For this review, take the finished solid that the model builds, in its own axes (mm). Face numbers are marked on the shaded views. A direction names the side the tool comes from. Give positions to 0.01 mm unless a question says otherwise; leave off trailing zeros. Loops run counter-clockwise (first coordinate to the right, second up) from the corner with the lowest first, then second, coordinate; pieces in that order, holes last. Notation, with made-up numbers: (22.25, -18) -> (77.25, -18) arc R35 ccw to (77.25, 14) -> close; hole circle Ø4 at (-34, 48.25). An arc over 180 degrees is marked (long way). One line per question, with ' | ' between items. Start each with the question number.
(1) Consider section A-A (y = 11.5). Write out the cut boundary in (x, z), and give its area (3 significant figures).
(2) Wall thickness on probe 1 along Z at (x, y) = (53.5, -22); probe 2 along Z at (x, y) = (6, -6.5): over which ranges is each line inside the solid? List them lowest first.
(3) Tool access review of the marked faces 1 and 2: name each direction out of +Z, -Z, +X, -X, +Y, -Y from which nothing blocks a thin tool from reaching the whole face with its end or side.
(4) Consider section B-B (z = 31.5). Write out the cut boundary in (x, y).
(5) Consider section C-C (x = 35.5). Write out the cut boundary in (y, z), and give its area (3 significant figures).
(6) Insertion check: P1, Ø4, axis at y = -8.5, z = 45, coming from the -X side. The pin has a flat end and moves straight along its axis. Give the tip position at first contact, or say it passes through.
from build123d import *

# Parameters (mm, degrees)
F0_W          = 76.2
F0_H          = 50.8
F1_DEPTH      = 25.4
F3_DEPTH      = 25.4
F4_W          = 50.8
F4_H          = 25.4
F5_DEPTH      = 25.4
F5_DEPTH_BACK = 87.34144


with BuildPart() as f1:
    # F0 (on Front) → F1 (new body, symmetric)
    with BuildSketch(Plane.XZ):
        with Locations((38.1, 25.4)):
            Rectangle(F0_W, F0_H)
    extrude(amount=F1_DEPTH, both=True)

    # F2 (on Front) → F3 (cut, symmetric)
    with BuildSketch(Plane.XZ):
        Polygon((0, 50.8), (0, 38.1), (12.7, 50.8), align=None)
    extrude(amount=F3_DEPTH, both=True, mode=Mode.SUBTRACT)

    # F4 (on Front) → F5 (cut, two sides)
    with BuildSketch(Plane.XZ) as f5_sk:
        with Locations((50.8, 38.1)):
            Rectangle(F4_W, F4_H)
    extrude(amount=F5_DEPTH, mode=Mode.SUBTRACT)
    extrude(f5_sk.sketch, amount=-F5_DEPTH_BACK, mode=Mode.SUBTRACT)


solid = f1.part
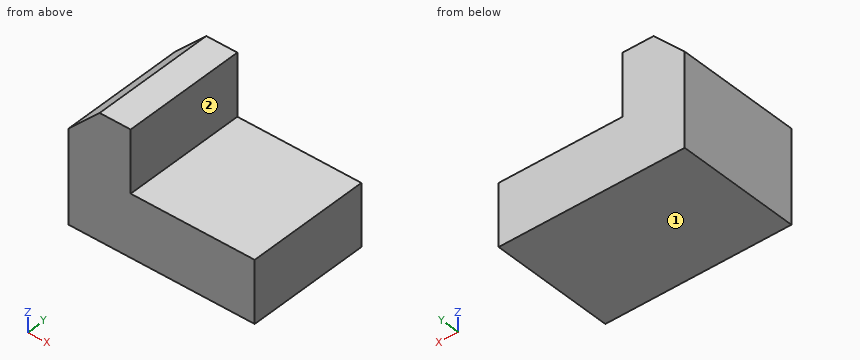
A:
1) outline: (0, 0) -> (76.2, 0) -> (76.2, 25.4) -> (25.4, 25.4) -> (25.4, 50.8) -> (12.7, 50.8) -> (0, 38.1) -> close | area: 2,500 mm^2
2) probe 1: z = 0 to 25.4 | probe 2: z = 0 to 44.1
3) face 1: -Z, +X, -X, +Y, -Y | face 2: +Z, +X, +Y, -Y
4) outline: (0, -25.4) -> (25.4, -25.4) -> (25.4, 25.4) -> (0, 25.4) -> close
5) outline: (-25.4, 0) -> (25.4, 0) -> (25.4, 25.4) -> (-25.4, 25.4) -> close | area: 1,290 mm^2
6) P1: stops at x = 4.9
